from build123d import *

# Parameters (mm, degrees)
BOSS_EXTRUDE1_DEPTH = 25
SKETCH2_R           = 3.05
BOSS_EXTRUDE2_DEPTH = 1.6
SKETCH3_R           = 1
BOSS_EXTRUDE3_DEPTH = 5.6
SKETCH4_R           = 4.95
BOSS_EXTRUDE4_DEPTH = 2.3
BOSS_EXTRUDE5_START = 1.5
SKETCH5_R           = 1
BOSS_EXTRUDE5_DEPTH = 1.5
SKETCH6_W           = 8.4
SKETCH6_H           = 5
BOSS_EXTRUDE6_DEPTH = 1.6
FILLET1_R           = 1


with BuildPart() as part:
    # Sketch1 → Boss-Extrude1 (new body)
    with BuildSketch(Plane(origin=(0, 0, 0), x_dir=(1, 0, 0), z_dir=(0, 1, 0))):
        with BuildLine():
            Line((6.557247898, 7.55), (-6.557247898, 7.55))
            ThreePointArc((-6.557247898, 7.55), (-10, 0), (-6.557247898, -7.55))
            Line((-6.557247898, -7.55), (6.557247898, -7.55))
            ThreePointArc((6.557247898, -7.55), (9.098694384, -4.148946916), (10, 0))
            ThreePointArc((10, 0), (9.098694384, 4.148946916), (6.557247898, 7.55))
        make_face()
    extrude(amount=BOSS_EXTRUDE1_DEPTH)

    # Sketch2 → Boss-Extrude2 (add)
    with BuildSketch(Plane(origin=(0, 25, 0), x_dir=(1, 0, 0), z_dir=(0, 1, 0))):
        with Locations(Location((0, 0, 0), (0, 0, 270))):
            Circle(SKETCH2_R)
    extrude(amount=BOSS_EXTRUDE2_DEPTH)

    # Sketch3 → Boss-Extrude3 (add)
    with BuildSketch(Plane(origin=(0, 26.6, 0), x_dir=(1, 0, 0), z_dir=(0, 1, 0))):
        with Locations(Location((0, 0, 0), (0, 0, 270))):
            Circle(SKETCH3_R)
    extrude(amount=BOSS_EXTRUDE3_DEPTH)

    # Sketch4 → Boss-Extrude4 (add)
    with BuildSketch(Plane.XZ):
        with Locations(Location((0, 0, 0), (0, 0, 270))):
            Circle(SKETCH4_R)
    extrude(amount=BOSS_EXTRUDE4_DEPTH)

    # Sketch5 → Boss-Extrude5 (add)
    with BuildSketch(Plane.XZ.offset(2.3).offset(BOSS_EXTRUDE5_START)):
        with Locations(Location((0, 0, 0), (0, 0, 90))):
            Circle(SKETCH5_R)
    extrude(amount=-BOSS_EXTRUDE5_DEPTH)

    # Sketch6 → Boss-Extrude6 (add)
    with BuildSketch(Plane.XY.offset(7.55)):
        with Locations((0, 2.5)):
            Rectangle(SKETCH6_W, SKETCH6_H)
    extrude(amount=BOSS_EXTRUDE6_DEPTH)

    # Fillet1
    fillet1_edges = [part.edges().sort_by_distance(p)[0] for p in [
        (-4.2, 2.5, 9.15),
        (0, 0, 9.15),
        (4.2, 2.5, 9.15),
    ]]
    fillet(fillet1_edges, radius=FILLET1_R)


solid = part.part
Part model, mm, in its own coordinate system. A direction names the side the tool comes from. Give positions to 0.01 mm unless a question says otherwise; leave off trailing zeros. Loops run counter-clockwise (first coordinate to the right, second up) from the corner with the lowest first, then second, coordinate; pieces in that order, holes last. Notation, with made-up numbers: (66.5, 0.25) -> (71.5, 0.25) arc R25 cw to (71.5, 28.25) -> close; hole circle Ø9 at (75.25, -17.75). An arc over 180 degrees is marked (long way). Write each question's results on one line, items separated by ' | '. Start each with the question number.
Q1. Wall check: L1, parallel to Y at x = -4.25, z = 0.5; L2, parallel to Y at x = -1, z = 6.25; L3, parallel to Z at x = -2.5, y = 22.5. Give the ranges that are in metal, low to high.
Q2. Band-saw the part on B-B on z = 1.5. List the corners of the cut face in (x, y).
Q3. Band-saw the part on C-C on y = 21. List the corners of the cut face in (x, z).
Q4. Pin check, flat tips, straight feed: P1, Ø3, axis at x = -5.5, y = 16.5, coming from the +Z side; P2, Ø2, axis at y = 10.5, z = 2.5, coming from the -X side; P3, Ø0.7, axis at y = 3, z = 7.5, coming from the +X side. Stop position of each tip, or through.
Q5. Band-saw the part on D-D on x = 0. List the corners of the cut face in (y, z).
Q6. Band-saw the part on A-A on x = 2. List the corners of the cut face in (y, z), plus the area to 3 significant figures.
Q7. Which spindle directions (+Z, -Z, +X, -X, +Y, -Y) get a long thin tool onto all of the face, cutting with end or side? Do faces 1 (the face through (0, 5, 8)), 2 (the face through (-1, 29, 0)), 3 (the face through (1.49, -1.13, -4.72)). Say none if no direction does.
Results are:
1) L1: y = -2.3 to 25 | L2: y = 0 to 25 | L3: z = -7.55 to 7.55
2) outline: (-9.89, 0) -> (-4.72, 0) -> (-4.72, -2.3) -> (4.72, -2.3) -> (4.72, 0) -> (9.89, 0) -> (9.89, 25) -> (2.66, 25) -> (2.66, 26.6) -> (-2.66, 26.6) -> (-2.66, 25) -> (-9.89, 25) -> close
3) outline: (-6.56, -7.55) -> (6.56, -7.55) arc R10 ccw to (6.56, 7.55) -> (-6.56, 7.55) arc R10 ccw to start
4) P1: stops at z = 7.55 | P2: stops at x = -9.89 | P3: stops at x = 6.99
5) outline: (-3.8, -1) -> (-2.3, -1) -> (-2.3, -4.95) -> (0, -4.95) -> (0, -7.55) -> (25, -7.55) -> (25, -3.05) -> (26.6, -3.05) -> (26.6, -1) -> (32.2, -1) -> (32.2, 1) -> (26.6, 1) -> (26.6, 3.05) -> (25, 3.05) -> (25, 7.55) -> (5, 7.55) -> (5, 9.15) -> (1, 9.15) arc R1 ccw to (0, 8.15) -> (0, 4.95) -> (-2.3, 4.95) -> (-2.3, 1) -> (-3.8, 1) -> close
6) outline: (-2.3, -4.53) -> (0, -4.53) -> (0, -7.55) -> (25, -7.55) -> (25, -2.3) -> (26.6, -2.3) -> (26.6, 2.3) -> (25, 2.3) -> (25, 7.55) -> (5, 7.55) -> (5, 9.15) -> (1, 9.15) arc R1 ccw to (0, 8.15) -> (0, 4.53) -> (-2.3, 4.53) -> close | area: 413 mm²
7) face 1: +Z, +X, -X, +Y | face 2: +Y | face 3: -Y
